```python
from build123d import *

# Parameters (mm, degrees)
SKETCH1_W          = 60
SKETCH1_H          = 10
SKETCH2_R          = 8
CUT_EXTRUDE1_DEPTH = 171
CIRPATTERN1_COUNT  = 8


with BuildPart() as part:
    # Sketch1 → Revolve1 (revolve)
    with BuildSketch(Plane.XY, mode=Mode.PRIVATE) as revolve1_sk:
        with BuildLine():
            ThreePointArc((75, 31.286171589), (71.464466094, 29.821705495), (70, 26.286171589))
            Line((70, 26.286171589), (70, 21.286171589))
            Line((70, 21.286171589), (60, 21.286171589))
            Line((60, 21.286171589), (60, 36.286171589))
            Line((60, 36.286171589), (65, 36.286171589))
            Line((65, 36.286171589), (65, 41.286171589))
            Line((65, 41.286171589), (120, 41.286171589))
            Line((120, 41.286171589), (120, 31.286171589))
            Line((120, 31.286171589), (75, 31.286171589))
        make_face()
        with Locations((30, 26.286171589)):
            Rectangle(SKETCH1_W, SKETCH1_H)
    revolve(revolve1_sk.sketch.rotate(Axis((0, 97.731625762, 0), (0, -1, 0)), 90), axis=Axis((0, 97.731625762, 0), (0, -1, 0)))

    # Sketch2 → Cut-Extrude1 (cut, through all)
    with BuildSketch(Plane.XZ.offset(-31.286171589)):
        with Locations(Location((79.233979131, 46.754428144, 0), (0, 0, 270))):
            Circle(SKETCH2_R)
    cut_extrude1 = extrude(amount=-CUT_EXTRUDE1_DEPTH, mode=Mode.SUBTRACT)

    # CirPattern1: Cut-Extrude1 ×8 about axis
    cirpattern1_axis = Axis((0, 0, 0), (0, 1, 0))
    for i in range(1, CIRPATTERN1_COUNT):
        add(cut_extrude1.rotate(cirpattern1_axis, i * 360 / CIRPATTERN1_COUNT), mode=Mode.SUBTRACT)


solid = part.part
```
Work out the finished part from the listing and answer in its coordinate system (mm). A direction names the side the tool comes from. Round coordinates to 2 decimals unless told otherwise and drop trailing zeros. Write each loop counter-clockwise with the first axis right and the second up, starting at its lowest first coordinate (ties: lowest second). Pieces come first, ordered by that corner, then holes. Notation, with made-up numbers: (39.5, 36) -> (98.5, 36) arc R18 ccw to (98.5, 58) -> close; hole circle Ø6 at (35, 62.5). An arc over 180 degrees is marked (long way). Write each question's results on one line, items separated by ' | '.
1) Consider line 1 along Z through (x, y) = (-25, 36); line 2 along X through (y, z) = (37, 21); line 3 along X through (y, z) = (36.5, -83.5). Determine where each line is inside the solid, lowest interval first. Write a range as [from, to].
Findings:
line 1: z = [-117.37, -96.82], [-81.35, -54.54], [54.54, 117.37] | line 2: x = [-118.15, -96.84], [-81.33, -61.51], [61.51, 118.15] | line 3: x = [-86.18, -28.69], [-17.24, 39.99], [53.52, 86.18]
2) Which of the six approach directions +Z, -Z, +X, -X, +Y, -Y give full straight-line access (tool end or side, diameter ignored) to faces 4 (the cylindrical face through (-50.59, 33.82, 32.26)), 5 (the flat face through (-55, 31.286, 52)), 6 (the cylindrical face through (26.025, 36.216, 81.695))?
Findings:
face 4: +Y | face 5: -Y | face 6: +Y, -Y
3) For a pull along X with two mould halves and no side action, classify faces 1 (the cylindrical face through (71.424, 36.216, 48.489)), 2 (the flat face through (-1, 21.286, 1)), 3 (the cylindrical face through (68.335, 23.751, -15.175)) as +X half, -X half, draft (parallel to the pull), parting line (faces both ways), or undercut.
Findings:
face 1: undercut | face 2: draft | face 3: parting line
4) The part is cut by section B-B (x = 0). Write down the section's boundary in (y, z).
Findings:
outline: (21.29, -70) -> (26.29, -70) arc R5 cw to (31.29, -75) -> (31.29, -120) -> (41.29, -120) -> (41.29, -65) -> (36.29, -65) -> (36.29, -60) -> (31.29, -60) -> (31.29, 60) -> (36.29, 60) -> (36.29, 65) -> (41.29, 65) -> (41.29, 120) -> (31.29, 120) -> (31.29, 75) arc R5 cw to (26.29, 70) -> (21.29, 70) -> close
5) The part is cut by section A-A (z = 0). Write down the section's boundary in (x, y).
Findings:
outline: (-120, 31.29) -> (-75, 31.29) arc R5 cw to (-70, 26.29) -> (-70, 21.29) -> (70, 21.29) -> (70, 26.29) arc R5 cw to (75, 31.29) -> (120, 31.29) -> (120, 41.29) -> (65, 41.29) -> (65, 36.29) -> (60, 36.29) -> (60, 31.29) -> (-60, 31.29) -> (-60, 36.29) -> (-65, 36.29) -> (-65, 41.29) -> (-120, 41.29) -> close
6) Flat-ended cylindrical pins translate along their axes: pin 1 (1 mm diameter, centred on y = 33.5, z = -64.5, fed in from +X); pin 2 (1.5 mm diameter, centred on x = -19, z = 10.5, fed in from +Y); pin 3 (21 mm diameter, centred on x = 46.75, z = -79.23, fed in from -Y). Find the tip coordinate at first contact, or state that the pin passes through.
Findings:
pin 1: stops at x = 101.51 | pin 2: stops at y = 31.29 | pin 3: stops at y = 31.29
